Here's how the part is built. I have some questions about the finished solid (model axes, mm). A direction names the side the tool comes from. Round coordinates to 2 decimals unless told otherwise and drop trailing zeros. Write each loop counter-clockwise with the first axis right and the second up, starting at its lowest first coordinate (ties: lowest second). Pieces come first, ordered by that corner, then holes. Notation, with made-up numbers: M 1.5,-18 L 47.5,-18 A32 ccw 47.5,13 Z; hole C 22,-12 d7. An arc over 180 degrees is marked long. Use a Markdown table: item, result. Add a question column.
```python
from build123d import *

# Parameters (mm, degrees)
SKETCH1_W           = 139.7
SKETCH1_H           = 82.55
BOSS_EXTRUDE1_DEPTH = 6.35
SKETCH2_W           = 12.7
SKETCH2_H           = 6.35
BOSS_EXTRUDE2_DEPTH = 6.35
CUT_EXTRUDE1_DEPTH  = 6.35
CUT_EXTRUDE8_DEPTH  = 6.35
CUT_EXTRUDE2_DEPTH  = 6.35
SKETCH5_R           = 6.254
SKETCH5_R_2         = 1.504
CUT_EXTRUDE9_DEPTH  = 6.35


with BuildPart() as part:
    # Sketch1 → Boss-Extrude1 (new body)
    with BuildSketch(Plane.XY):
        Rectangle(SKETCH1_W, SKETCH1_H)
    extrude(amount=BOSS_EXTRUDE1_DEPTH)

    # Sketch2 → Boss-Extrude2 (add)
    with BuildSketch(Plane(origin=(0, 0, 0), x_dir=(-1, 0, 0), z_dir=(0, 0, -1))):
        with Locations((-63.5, -44.45)):
            Rectangle(SKETCH2_W, SKETCH2_H)
        with Locations((-25.4, 44.45)):
            Rectangle(SKETCH2_W, SKETCH2_H)
    boss_extrude2 = extrude(amount=-BOSS_EXTRUDE2_DEPTH)

    # Sketch3 → Cut-Extrude1 (cut)
    with BuildSketch(Plane(origin=(0, 0, 0), x_dir=(-1, 0, 0), z_dir=(0, 0, -1))):
        Polygon((-52.9336, -41.275), (-52.9336, -32.512), (-55.245, -32.512), (-55.245, -29.337), (-52.9336, -29.337), (-52.9336, -26.035), (-48.6664, -26.035), (-48.6664, -29.337), (-46.355, -29.337), (-46.355, -32.512), (-48.6664, -32.512), (-48.6664, -41.275), align=None)
    cut_extrude1 = extrude(amount=-CUT_EXTRUDE1_DEPTH, mode=Mode.SUBTRACT)

    # Sketch7 → Cut-Extrude8 (cut)
    with BuildSketch(Plane(origin=(0, 0, 0), x_dir=(-1, 0, 0), z_dir=(0, 0, -1))):
        Polygon((-38.1, 41.275), (-69.85, -34.925), (-69.85, 41.275), align=None)
    cut_extrude8 = extrude(amount=-CUT_EXTRUDE8_DEPTH, mode=Mode.SUBTRACT)

    # Mirror2: Boss-Extrude2, Cut-Extrude8 across plane
    add(boss_extrude2.mirror(Plane(origin=(0, 0, 0), x_dir=(0, 0, 1), z_dir=(1, 0, 0))))
    add(cut_extrude8.mirror(Plane(origin=(0, 0, 0), x_dir=(0, 0, 1), z_dir=(1, 0, 0))), mode=Mode.SUBTRACT)

    # Mirror4: Cut-Extrude1 across plane
    add(cut_extrude1.mirror(Plane(origin=(0, 0, 0), x_dir=(0, 0, 1), z_dir=(1, 0, 0))), mode=Mode.SUBTRACT)

    # Sketch4 → Cut-Extrude2 (cut)
    with BuildSketch(Plane(origin=(0, 0, 0), x_dir=(-1, 0, 0), z_dir=(0, 0, -1))):
        Polygon((2.1209, 41.275), (-2.1209, 41.275), (-2.1209, 32.512), (-4.445, 32.512), (-4.445, 29.337), (-2.1209, 29.337), (-2.1209, 26.035), (2.1209, 26.035), (2.1209, 29.337), (4.445, 29.337), (4.445, 32.512), (2.1209, 32.512), align=None)
    extrude(amount=-CUT_EXTRUDE2_DEPTH, mode=Mode.SUBTRACT)

    # Sketch5 → Cut-Extrude9 (cut)
    with BuildSketch(Plane(origin=(0, 0, 0), x_dir=(-1, 0, 0), z_dir=(0, 0, -1))):
        with Locations((0, -26.7)):
            Circle(SKETCH5_R)
        with Locations((-15.5, -19.7)):
            Circle(SKETCH5_R_2)
        with Locations((-7.75, -6.276606241)):
            Circle(SKETCH5_R_2)
        with Locations((7.75, -6.276606241)):
            Circle(SKETCH5_R_2)
        with Locations((15.5, -19.7)):
            Circle(SKETCH5_R_2)
        with Locations((7.75, -33.123393759)):
            Circle(SKETCH5_R_2)
        with Locations((-7.75, -33.123393759)):
            Circle(SKETCH5_R_2)
    extrude(amount=-CUT_EXTRUDE9_DEPTH, mode=Mode.SUBTRACT)


solid = part.part
```
Item 1: Imagine slicing it at B-B on x = -15.5. List the corners of the cut face in (y, z) for me (3 decimals).
Item 2: For pin 1 Ø3.5 at (y, z) = (31, 2) entering from -X; pin 2 Ø3 at (y, z) = (45.5, 3.5) entering from +X; pin 3 Ø2.5 at (y, z) = (-27, 2) entering from +X, each with a flat end and sliding along its axis, tell me the tip position at first contact or that it passes through.
Item 3: Imagine slicing it at D-D on x = 44. List the corners of the cut face in (y, z) for me (3 decimals), plus the area to 3 significant figures.
Item 4: Imagine slicing it at C-C on z = 2.75. Count the separate pieces of the cut face and the enclosed holes in it, plus the area to 3 significant figures.
Item 5: If we mould it in two halves opening along Y, with no side actions, what happens to faces 1 (the face through (52.934, -37, 3)), 2 (the face through (51, -26.035, 3)), 3 (the face through (-4.445, 31, 3))? For each: +Y half, -Y half, draft (parallel to the pull), parting line (faces both ways), or undercut.
Item 6: I need wall thicknesses on probe 1 along X at (y, z) = (-7.5, 1.5); probe 2 along X at (y, z) = (-42.5, 4.5); probe 3 along Y at (x, z) = (15.5, 2) (3 decimals). Which ranges of each line are inside material? Lowest first, please. Write a range as from..to.
Item 7: On a 3-axis mill with a long thin cutter (end or side, diameter ignored), from which of +Z, -Z, +X, -X, +Y, -Y can I reach the whole of each face in a straight line? I mean faces 4 (the face through (57.15, -44, 3)), 5 (the face through (31.75, 44, 3)), 6 (the face through (10, 41.275, 3)). Say none if no direction works.
Item 8: Imagine slicing it at A-A on x = 0. List the corners of the cut face in (y, z) for me (3 decimals), plus the area to 3 significant figures.
The answers:
| question | item | result |
|---|---|---|
| 1 | outline | M -41.275,0 L -21.204,0 L -21.204,6.35 L -41.275,6.35 Z; M -18.196,0 L 41.275,0 L 41.275,6.35 L -18.196,6.35 Z |
| 2 | pin 1 | x = -43.11 |
| 2 | pin 2 | x = 31.75 |
| 2 | pin 3 | x = 67.07 |
| 3 | outline | M -41.275,0 L 27.115,0 L 27.115,6.35 L -41.275,6.35 Z |
| 3 | area | 434 mm² |
| 4 | separate pieces | 1 |
| 4 | enclosed holes | 7 |
| 4 | area | 9,030 mm² |
| 5 | face 1 | draft |
| 5 | face 2 | -Y half |
| 5 | face 3 | undercut |
| 6 | probe 1 | -58.42..-8.62, -6.88..6.88, 8.62..58.42 |
| 6 | probe 2 | -69.85..-57.15, 57.15..69.85 |
| 6 | probe 3 | -41.275..-21.204, -18.196..41.275 |
| 7 | face 4 | +Z, -Z, -Y |
| 7 | face 5 | +Z, -Z, +X, +Y |
| 7 | face 6 | +Z, -Z, +Y |
| 8 | outline | M -41.275,0 L -32.954,0 L -32.954,6.35 L -41.275,6.35 Z; M -20.446,0 L 26.035,0 L 26.035,6.35 L -20.446,6.35 Z |
| 8 | area | 348 mm² |
